from build123d import *

# Parameters (mm, degrees)
F1_DEPTH = 20
F2_R     = 2.5
F3_DEPTH = 25
F4_R     = 2.5
F5_DEPTH = 25


with BuildPart() as f1:
    # F0 (on Front) → F1 (new body, symmetric)
    with BuildSketch(Plane.XZ):
        Polygon((-60, 2.5), (-60, 0), (0, 0), (0, 60), (-2.5, 60), (-2.5, 2.5), align=None)
    extrude(amount=F1_DEPTH, both=True)

    # F2 (on face) → F3 (cut)
    with BuildSketch(Plane(origin=(-2.5, 0, 0), x_dir=(0, -1, 0), z_dir=(-1, 0, 0))):
        with Locations((0, 31.25)):
            Circle(F2_R)
        with Locations((-14, 8.5)):
            Circle(F2_R)
        with Locations((-14, 54)):
            Circle(F2_R)
        with Locations((14, 54)):
            Circle(F2_R)
        with Locations((14, 8.5)):
            Circle(F2_R)
    extrude(amount=-F3_DEPTH, mode=Mode.SUBTRACT)

    # F4 (on face) → F5 (cut)
    with BuildSketch(Plane.XY.offset(2.5)):
        with Locations((-54, 0)):
            Circle(F4_R)
        with Locations((-31.25, 14)):
            Circle(F4_R)
        with Locations((-31.25, -14)):
            Circle(F4_R)
        with Locations((-8.5, 0)):
            Circle(F4_R)
    extrude(amount=-F5_DEPTH, mode=Mode.SUBTRACT)


solid = f1.part
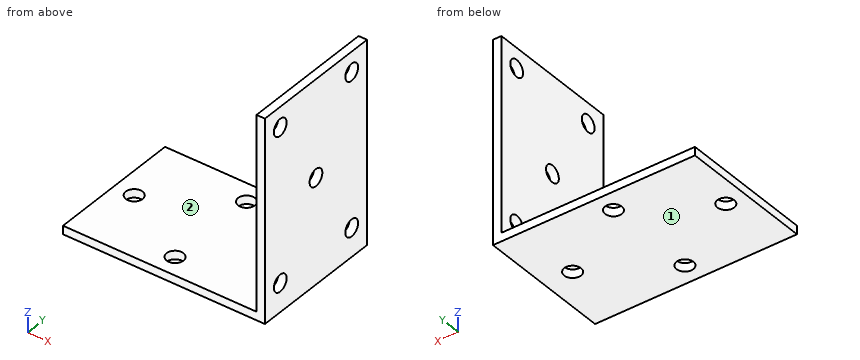
Can you work these out from the model? Positions are in its coordinate system, mm. Face numbers are marked on the shaded views. A direction names the side the tool comes from. Round coordinates to 2 decimals unless told otherwise and drop trailing zeros. Write each loop counter-clockwise with the first axis right and the second up, starting at its lowest first coordinate (ties: lowest second). Pieces come first, ordered by that corner, then holes. Notation, with made-up numbers: (57, 0.5) - (81, 0.5) arc R19 ccw to (81, 13.5) - close; hole circle Ø11 at (21.5, -12). An arc over 180 degrees is marked (long way). Write each question's results on one line, items separated by ' | '. Start each with the question number.
1) Which directions (+Z, -Z, +X, -X, +Y, -Y) give clear straight access to the entire face, cutting with the end or side of a thin tool? Please do the marked faces 1 and 2.
2) Suppose I cut it at D-D (z = 54). List the corners of the cut face in (x, y) for me, and give its area (3 significant figures).
3) For pin 1 Ø12 at (y, z) = (-4.5, 48) entering from -X; pin 2 Ø8 at (x, y) = (-31.25, -14) entering from +Z, each with a flat end and sliding along its axis, tell me the tip position at first contact or that it passes through.
4) Please list where these lines run through material, in increasing order: line 1 (Y direction, x = -31.25, z = 1.8); line 2 (Z direction, x = -1, y = 14); line 3 (Y direction, x = -1, z = 8).
5) Suppose I cut it at A-A (x = -8.5). List the corners of the cut face in (y, z) for me, and give its area (3 significant figures).
6) Suppose I cut it at C-C (y = 14). List the corners of the cut face in (x, z) for me.
7) Suppose I cut it at B-B (z = 31.25). List the corners of the cut face in (x, y) for me, and give its area (3 significant figures).
Here are the results:
1) face 1: -Z, +X, -X, +Y, -Y | face 2: +Z, -X, +Y, -Y
2) outline: (-2.5, -20) - (0, -20) - (0, -16.5) - (-2.5, -16.5) - close; (-2.5, -11.5) - (0, -11.5) - (0, 11.5) - (-2.5, 11.5) - close; (-2.5, 16.5) - (0, 16.5) - (0, 20) - (-2.5, 20) - close | area: 75.0 mm2
3) pin 1: stops at x = -2.5 | pin 2: stops at z = 2.5
4) line 1: y = -20 to -16.5, -11.5 to 11.5, 16.5 to 20 | line 2: z = 0 to 6, 11 to 51.5, 56.5 to 60 | line 3: y = -20 to -16.45, -11.55 to 11.55, 16.45 to 20
5) outline: (-20, 0) - (-2.5, 0) - (-2.5, 2.5) - (-20, 2.5) - close; (2.5, 0) - (20, 0) - (20, 2.5) - (2.5, 2.5) - close | area: 87.5 mm2
6) outline: (-60, 0) - (-33.75, 0) - (-33.75, 2.5) - (-60, 2.5) - close; (-28.75, 0) - (0, 0) - (0, 6) - (-2.5, 6) - (-2.5, 2.5) - (-28.75, 2.5) - close; (-2.5, 11) - (0, 11) - (0, 51.5) - (-2.5, 51.5) - close; (-2.5, 56.5) - (0, 56.5) - (0, 60) - (-2.5, 60) - close
7) outline: (-2.5, -20) - (0, -20) - (0, -2.5) - (-2.5, -2.5) - close; (-2.5, 2.5) - (0, 2.5) - (0, 20) - (-2.5, 20) - close | area: 87.5 mm2
